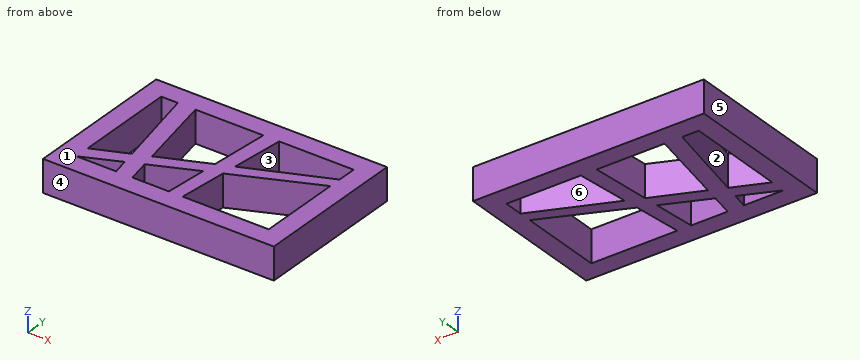
```python
from build123d import *

# Parameters (mm, degrees)
F0_W     = 180
F0_H     = 120
F1_DEPTH = 25


with BuildPart() as f1:
    # F0 (on Top) → F1 (new body)
    with BuildSketch(Plane.XY):
        Rectangle(F0_W, F0_H)
        Polygon((-46.476726, -32.595648), (-43.98147, -45), (-75, -45), align=None, mode=Mode.SUBTRACT)
        Polygon((-0.156685, -12.451744), (-2.835166, -45), (-31.363267, -45), (-34.676992, -27.464117), align=None, mode=Mode.SUBTRACT)
        Polygon((75, 20.232793), (75, -45), (7.862872, -45), (11.653141, -7.315824), align=None, mode=Mode.SUBTRACT)
        Polygon((-75, -32.983091), (-75, 45), (-62.085841, 45), (-48.629935, -21.891666), align=None, mode=Mode.SUBTRACT)
        Polygon((-36.67982, -16.865368), (-48.37041, 45), (4.571168, 45), (0.776578, -1.110959), align=None, mode=Mode.SUBTRACT)
        Polygon((16.915059, 45), (75, 45), (75, 30.107906), (12.785247, 3.939967), align=None, mode=Mode.SUBTRACT)
    extrude(amount=F1_DEPTH)


solid = f1.part
```
Part model, mm, in its own coordinate system. Face numbers are marked on the shaded views. A direction names the side the tool comes from. Coordinates: 2 decimals unless noted, no trailing zeros. Order: outer loops, then holes, each group sorted by start corner. A loop starts at its lowest first (then second) coordinate and runs counter-clockwise, first axis right, second up. Notation, with made-up numbers: (-1, -6) -> (14, -6) arc R17 cw to (14, 16) -> close; hole circle Ø5 at (26.5, 38). An arc over 180 degrees is marked (long way). Put each result on its own line as item: value. Start each with the question number.
(1) Mould opens along Y. For the marked faces 1, 2, 3 and 4 say: pulls with the +Y half, pulls with the -Y half, needs draft (parallel to the pull), parting line crosses it, or undercut.
(2) Band-saw the part on A-A (x = -54.5). Give the cut face in (y, z), then the cut area to 3 significant figures.
(3) Which spindle directions (+Z, -Z, +X, -X, +Y, -Y) get a long thin tool onto all of the face, cutting with end or side? Do the marked faces 5 and 6. Say none if no direction does.
(4) Pin check, flat tip, straight feed: pin 1 Ø6 at (x, y) = (-15.5, 40.5) entering from -Z. Stop position of the tip, or through.
(5) Band-saw the part on D-D (y = 16). Give the cut face in (x, z), then the cut area to 3 significant figures.
(6) Probe line 1 along Y through (x, z) = (44, 1.75); line 2 along Y through (x, z) = (24.5, 20.75); line 3 along X through (y, z) = (44.5, 4.75). List the from-to ranges inside material, lowest first. Write a range as [from, to].
(7) Band-saw the part on B-B (y = -43). Give the cut face in (x, z).
(8) Band-saw the part on C-C (z = 18.5). Give the cut face in (x, y), then the cut area to 3 significant figures.
Determined:
1. face 1: needs draft
1. face 2: undercut
1. face 3: undercut
1. face 4: pulls with the -Y half
2. outline: (-60, 0) -> (-45, 0) -> (-45, 25) -> (-60, 25) -> close; (-36.08, 0) -> (-24.36, 0) -> (-24.36, 25) -> (-36.08, 25) -> close; (7.29, 0) -> (60, 0) -> (60, 25) -> (7.29, 25) -> close
2. area: 1,990 mm²
3. face 5: +Z, -Z, -X, +Y, -Y
3. face 6: +Z, -Z
4. pin 1: passes through
5. outline: (-90, 0) -> (-75, 0) -> (-75, 25) -> (-90, 25) -> close; (-56.25, 0) -> (-42.89, 0) -> (-42.89, 25) -> (-56.25, 25) -> close; (2.18, 0) -> (14, 0) -> (14, 25) -> (2.18, 25) -> close; (41.46, 0) -> (65.27, 0) -> (65.27, 25) -> (41.46, 25) -> close; (75, 0) -> (90, 0) -> (90, 25) -> (75, 25) -> close
5. area: 1,970 mm²
6. line 1: y = [-60, -45], [6.75, 17.07], [45, 60]
6. line 2: y = [-60, -45], [-1.73, 8.87], [45, 60]
6. line 3: x = [-90, -75], [-61.99, -48.28], [4.53, 16.86], [75, 90]
7. outline: (-90, 0) -> (-70.4, 0) -> (-70.4, 25) -> (-90, 25) -> close; (-44.38, 0) -> (-31.74, 0) -> (-31.74, 25) -> (-44.38, 25) -> close; (-2.67, 0) -> (8.06, 0) -> (8.06, 25) -> (-2.67, 25) -> close; (75, 0) -> (90, 0) -> (90, 25) -> (75, 25) -> close
8. outline: (-90, -60) -> (90, -60) -> (90, 60) -> (-90, 60) -> close; hole (-75, -45) -> (-43.98, -45) -> (-46.48, -32.6) -> close; hole (-75, -32.98) -> (-48.63, -21.89) -> (-62.09, 45) -> (-75, 45) -> close; hole (-48.37, 45) -> (-36.68, -16.87) -> (0.78, -1.11) -> (4.57, 45) -> close; hole (-34.68, -27.46) -> (-31.36, -45) -> (-2.84, -45) -> (-0.16, -12.45) -> close; hole (7.86, -45) -> (75, -45) -> (75, 20.23) -> (11.65, -7.32) -> close; hole (12.79, 3.94) -> (75, 30.11) -> (75, 45) -> (16.92, 45) -> close
8. area: 11,700 mm²
